from build123d import *

# Parameters (mm, degrees)
F1_DEPTH = 25
F5_DEPTH = 16.7
F8_DEPTH = 141.2028865991


with BuildPart() as f1:
    # F0 (on Right) → F1 (new body, symmetric)
    with BuildSketch(Plane.YZ):
        with BuildLine():
            Line((-36.5510998701, 0), (38.4489001299, 0))
            Line((38.4489001299, 0), (38.4489001299, 3))
            Line((38.4489001299, 3), (0.4813009491, 3))
            ThreePointArc((0.4813009491, 3), (-3.4854657523, 4.956192855), (-4.3483281823, 9.2940952255))
            Line((-4.3483281823, 9.2940952255), (28.8086734224, 133.0377098409))
            Line((28.8086734224, 133.0377098409), (12.6777121234, 137.3599878941))
            Line((12.6777121234, 137.3599878941), (-18.7688018566, 20))
            Line((-18.7688018566, 20), (-27.4621342932, 22.3293714059))
            Line((-27.4621342932, 22.3293714059), (-25.9092200226, 28.1249263637))
            Line((-25.9092200226, 28.1249263637), (-28.8069975014, 28.901383499))
            Line((-28.8069975014, 28.901383499), (-36.5510998701, 0))
        make_face()
    extrude(amount=F1_DEPTH, both=True)

    # F2 (on Right) → F3 (revolve, cut)
    with BuildSketch(Plane.YZ):
        with BuildLine():
            Line((12.2894835557, 135.9110991547), (0.6426265261, 92.4444369717))
            Line((0.6426265261, 92.4444369717), (13.8758103463, 88.8986160538))
            Line((13.8758103463, 88.8986160538), (23.8403435827, 126.0867603659))
            add(Edge.make_bspline(
                [(22.2214309345, 135.113339), (24.3902161666, 133.5995613693), (24.376132241, 128.0570148586), (23.8403435827, 126.0867603659)],
                knots=[0, 0, 0, 0, 9.1706052145, 9.1706052145, 9.1706052145, 9.1706052145], degree=3))
            add(Edge.make_bspline(
                [(12.2894835557, 135.9110991547), (16.0249762186, 136.7180167793), (20.3704343359, 135.803547418), (22.2214309345, 135.113339)],
                knots=[0, 0, 0, 0, 9.9639349657, 9.9639349657, 9.9639349657, 9.9639349657], degree=3))
        make_face()
    revolve(axis=Axis((0, 7.2592184362, 90.6715265127), (0, -0.9659258263, 0.2588190451)), mode=Mode.SUBTRACT)

    # F4 (on face) → F5 (cut, through all)
    with BuildSketch(Plane(origin=(0, -6.3805692325, 1.7096683731), x_dir=(-1, 0, 0), z_dir=(0, 0.9659258263, -0.2588190451))):
        with BuildLine():
            ThreePointArc((-25, 118.7396250955), (0, 127.9607931515), (25, 118.7396250955))
            Line((25, 118.7396250955), (25, 135.9607931515))
            Line((25, 135.9607931515), (-25, 135.9607931515))
            Line((-25, 135.9607931515), (-25, 118.7396250955))
        make_face()
    extrude(amount=-F5_DEPTH, mode=Mode.SUBTRACT)

    # F7 (on face) → F8 (cut, through all)
    with BuildSketch(Plane(origin=(0, -2.4484594232, -9.1377749675), x_dir=(1, 0, 0), z_dir=(0, 0.2588190451, 0.9659258263))):
        Polygon((-25, 37.1387856279), (-25, -35.3056513438), (-18.6619330295, 37.1387856279), align=None)
        Polygon((18.6619330295, 37.1387856279), (25, -35.3056513438), (25, 37.1387856279), align=None)
    extrude(amount=F8_DEPTH, mode=Mode.SUBTRACT)


solid = f1.part
Can you work these out from the model? Positions are in its coordinate system, mm. A direction names the side the tool comes from. Give positions to 0.01 mm unless a question says otherwise; leave off trailing zeros. Order: outer loops, then holes, each group sorted by start corner. A loop starts at its lowest first (then second) coordinate and runs counter-clockwise, first axis right, second up. Notation, with made-up numbers: M 57.5,-26 L 102.5,-26 A15 ccw 102.5,-5 Z; hole C 61,16 d4. An arc over 180 degrees is marked long. Use a Markdown table: item, result. Add a question column.
Item 1: Suppose I cut it at D-D (z = 17). List the corners of the cut face in (x, y) for me.
Item 2: Suppose I cut it at C-C (y = 9). List the corners of the cut face in (x, z) for me, then the cut area to 3 significant figures.
Item 3: If I drill on L1, parallel to Z at x = 10, y = 30; L2, parallel to Y at x = 8, z = 81; L3, parallel to Y at x = 17.5, z = 10, over which ranges is the centre line in solid material (lowest first)? Write a range as [from, to].
Item 4: Will these pins go through, and if not, where does the flat tip stop? pin 1 (1 mm diameter, centred on x = 13.5, z = 103.5, fed in from -Y); pin 2 (1 mm diameter, centred on y = 19.5, z = 111, fed in from -X); pin 3 (12 mm diameter, centred on y = 19, z = 82.5, fed in from +X).
Item 5: For faces 4 (the flat face through (0.346, -23.055, 21.148)), 5 (the flat face through (0.34, -14.99, 34.11)), 6 (the flat face through (0.315, 10.977, 66.49)), which set-ups out of +Z, -Z, +X, -X, +Y, -Y let a thin tool reach every point of the face, with its end or its side?
Item 6: Suppose I cut it at B-B (z = 116). List the corners of the cut face in (x, y) for me, then the cut area to 3 significant figures.
Item 7: We'd pull the mould along Y, two halves only. Please class faces 1 (the flat face through (0.35, -32.625, 14.653)), 2 (the flat face through (0, 20, 3)), 3 (the flat face through (0.346, -26.697, 25.187)): +Y half, -Y half, draft (parallel to the pull), parting line (faces both ways), or undercut.
Item 8: Suppose I cut it at A-A (y = 20). List the corners of the cut face in (x, z) for me, then the cut area to 3 significant figures.
Answer sheet:
| question | item | result |
|---|---|---|
| 1 | outline | M -25,-32 L 25,-32 L 22.49,-2.28 L -22.49,-2.28 Z |
| 2 | outline | M -22.75,70.7 L -22.49,59.11 L 22.49,59.11 L 22.75,70.7 Z; M -21.22,3 L -21.15,0 L 21.15,0 L 21.22,3 Z |
| 2 | area | 651 mm² |
| 3 | L1 | z = [0, 3] |
| 3 | L2 | y = [11.76, 14.87] |
| 3 | L3 | y = [-33.87, -4.16] |
| 4 | pin 1 | stops at y = 17.65 |
| 4 | pin 2 | stops at x = -22.75 |
| 4 | pin 3 | stops at x = 22.7 |
| 5 | face 4 | +X, -X |
| 5 | face 5 | +Z, +X, -X |
| 5 | face 6 | +X, -X, +Y |
| 6 | outline | M -22.75,21.14 L 22.75,21.14 L 22.49,24.24 L -22.49,24.24 Z |
| 6 | area | 141 mm² |
| 7 | face 1 | -Y half |
| 7 | face 2 | draft |
| 7 | face 3 | undercut |
| 8 | outline | M -22.75,111.75 L -22.49,100.16 L 22.49,100.16 L 22.75,111.75 Z; M -20.29,3 L -20.22,0 L 20.22,0 L 20.29,3 Z |
| 8 | area | 646 mm² |
